```python
from build123d import *

# Parameters (mm, degrees)
SKETCH1_R           = 3.5
BOSS_EXTRUDE1_DEPTH = 6.2
CHAMFER1_SIZE       = 1


with BuildPart() as part:
    # Sketch1 → Boss-Extrude1 (new body)
    with BuildSketch(Plane(origin=(0, 0, 0), x_dir=(1, 0, 0), z_dir=(0, 1, 0))):
        Polygon((6.4, -3.695041723), (6.4, 3.695041723), (0, 7.390083446), (-6.4, 3.695041723), (-6.4, -3.695041723), (0, -7.390083446), align=None)
        with Locations(Location((0, 0, 0), (0, 0, 90))):
            Circle(SKETCH1_R, mode=Mode.SUBTRACT)
    extrude(amount=BOSS_EXTRUDE1_DEPTH)

    # Chamfer1
    chamfer1_edges = [part.edges().sort_by_distance(p)[0] for p in [
        (3.2, 6.2, -5.542562584),
        (-3.2, 6.2, -5.542562584),
        (-6.4, 6.2, 0),
        (0, 0, 3.5),
        (0, 6.2, 3.5),
        (-3.2, 6.2, 5.542562584),
        (3.2, 6.2, 5.542562584),
        (-3.2, 0, 5.542562584),
        (-6.4, 0, 0),
        (-3.2, 0, -5.542562584),
        (6.4, 6.2, 0),
        (3.2, 0, -5.542562584),
        (6.4, 0, 0),
        (3.2, 0, 5.542562584),
    ]]
    chamfer(chamfer1_edges, length=CHAMFER1_SIZE)


solid = part.part
```
Geometry check sheet. Reference: the model listing, model coordinates, mm. Round coordinates to 2 decimals unless told otherwise and drop trailing zeros. Order: outer loops, then holes, each group sorted by start corner. A loop starts at its lowest first (then second) coordinate and runs counter-clockwise, first axis right, second up. Notation, with made-up numbers: (74.25, 42.5) -> (94.25, 42.5) arc R26 cw to (94.25, 56.5) -> close; hole circle Ø1 at (-21, -34.75). An arc over 180 degrees is marked (long way). Return JSON: item names as keys, results as strings. Group by question number.
Q1. Material ranges on probe 1 along X at (y, z) = (2.4, 0); probe 2 along X at (y, z) = (5.5, -2.5); probe 3 along Z at (x, y) = (-2, 0.5), recorded low to high. Write a range as from..to.
Q2. Section check A-A, the plane z = 0. Record the boundary of the cut face in (x, y).
Q3. Section check C-C, the plane x = 4.75. Record the boundary of the cut face in (y, z), plus the area to 3 significant figures.
Q4. Release check for a two-part mould opening along X. For faces 1 (the flat face through (5.9, 5.7, 0.1)), 2 (the cylindrical face through (3.417, 3.071, 0.759)), 3 (the flat face through (0, 0, 5)), 4 (the flat face through (-5.9, 0.5, -0.1)) record: released by +X, released by -X, zero draft, split by the parting line, or undercut.
Q5. Gauge pin test, flat ends, axial feed: pin 1 (4 mm diameter, centred on x = 0, z = 0, fed in from -Y); pin 2 (2 mm diameter, centred on x = -0.5, y = 3, fed in from -Z). Record the tip position at first contact, or that the pin passes through.
Q6. Section check B-B, the plane y = 2.75. Record the boundary of the cut face in (x, z).
Numbers:
{
 "1": {"probe 1": "-6.4..-3.5, 3.5..6.4", "probe 2": "-6.1..-2.86, 2.86..6.1", "probe 3": "-5.66..-3.46, 3.46..5.66"},
 "2": {"outline": "(-6.4, 1) -> (-5.4, 0) -> (-4.5, 0) -> (-3.5, 1) -> (-3.5, 5.2) -> (-4.5, 6.2) -> (-5.4, 6.2) -> (-6.4, 5.2) -> close; (3.5, 1) -> (4.5, 0) -> (5.4, 0) -> (6.4, 1) -> (6.4, 5.2) -> (5.4, 6.2) -> (4.5, 6.2) -> (3.5, 5.2) -> close"},
 "3": {"outline": "(0, -3.49) -> (1, -4.65) -> (5.2, -4.65) -> (6.2, -3.49) -> (6.2, 3.49) -> (5.2, 4.65) -> (1, 4.65) -> (0, 3.49) -> close", "area": "55.3 mm^2"},
 "4": {"face 1": "released by +X", "face 2": "undercut", "face 3": "zero draft", "face 4": "released by -X"},
 "5": {"pin 1": "through", "pin 2": "z = -7.39"},
 "6": {"outline": "(-6.4, -3.7) -> (0, -7.39) -> (6.4, -3.7) -> (6.4, 3.7) -> (0, 7.39) -> (-6.4, 3.7) -> close; hole circle Ø7 at (0, 0)"}
}
